Autodesk Inventor part; units mm, degrees
ref_plane "YZ Plane" through (0, 0, 0) normal (1, 0, 0) x (0, 1, 0)
ref_plane "XZ Plane" through (0, 0, 0) normal (0, 1, 0) x (-1, 0, 0)
ref_plane "XY Plane" through (0, 0, 0) normal (0, 0, 1) x (1, 0, 0)
sketch "Sketch1" plane through (0, 0, 0) normal (0, 0, 1) x (1, 0, 0)
  line L0 (-13.9879, -6.06) -> (16.0121, -6.06)
  line L1 (16.0121, -6.06) -> (16.0121, 23.94)
  line L2 (16.0121, 23.94) -> (-13.9879, 23.94)
  line L3 (-13.9879, 23.94) -> (-13.9879, -6.06)
  line L4 (-12.2879, 23.94) -> (-12.2879, -6.06)
  line L5 (-13.9879, -4.36) -> (16.0121, -4.36)
  line L6 (14.3121, -6.06) -> (14.3121, 23.94)
  line L7 (16.0121, 22.24) -> (-13.9879, 22.24)
  point P0 (0, 0)
  point P1 (14.3121, 22.24)
  point P2 (-12.2879, 22.24)
  point P3 (-12.2879, -4.36)
  point P4 (14.3121, -4.36)
  dimension "d1" = 30
  dimension "d3" = 1.7
  dimension "d4" = 1.7
  dimension "d5" = 1.7
  dimension "d6" = 1.7
extrude "Extrusion1" add sketch "Sketch1" against normal blind 129.75
extrude "Extrusion2" cut sketch "Sketch1" against normal blind 403 contours L4 L7 L6 L5
properties part number "Cablecanal Ranurado 30 x 30 L = 403" material "PVC-Piping"
Build history of the part. All positions in model axes, mm. A direction names the side the tool comes from. Give positions to 0.01 mm unless a question says otherwise; leave off trailing zeros. Order: outer loops, then holes, each group sorted by start corner. A loop starts at its lowest first (then second) coordinate and runs counter-clockwise, first axis right, second up. Notation, with made-up numbers: M 15,18.25 L 34,18.25 A25 ccw 34,55.25 Z; hole C 38.25,45 d10. An arc over 180 degrees is marked long. Write item = value, one per line. Start each with the question number.
(1) Probe L1, parallel to Y at x = -5, z = -81; L2, parallel to X at y = 10.25, z = -75.5. List the from-to ranges inside material, lowest first. Write a range as [from, to].
(2) Two-plate mould, pull along X, no slides. Class faces 1 (the flat face through (1, -4.36, -64)), 2 (the flat face through (1, -6.06, -64)), 3 (the flat face through (-13.988, 9, -64)), 4 (the flat face through (1, 22.24, -64)): released by +X, released by -X, zero draft, split by the parting line, or undercut.
(3) Slice it at B-B on y = 12.5. Write the cut outline in (x, z), plus the area to 3 significant figures.
(4) Which spindle directions (+Z, -Z, +X, -X, +Y, -Y) get a long thin tool onto all of the face, cutting with end or side? Do faces 5 (the flat face through (16.012, 9, -64)), 6 (the flat face through (-12.288, 9, -64)). Say none if no direction does.
(5) Slice it at C-C on x = 0.75. Write the cut outline in (y, z).
(6) Pin check, flat tip, straight feed: pin 1 Ø12 at (x, y) = (1, 18) entering from -Z. Stop position of the tip, or through.
(7) Slice it at A-A on z = -23. Write the cut outline in (x, y), plus the area to 3 significant figures.
Responses:
q1.L1 = [-6.06, -4.36], [22.24, 23.94]
q1.L2 = [-13.99, -12.29], [14.31, 16.01]
q2.face_1 = undercut
q2.face_2 = zero draft
q2.face_3 = released by -X
q2.face_4 = undercut
q3.outline = M -13.99,-129.75 L -12.29,-129.75 L -12.29,0 L -13.99,0 Z; M 14.31,-129.75 L 16.01,-129.75 L 16.01,0 L 14.31,0 Z
q3.area = 441 mm2
q4.face_5 = +Z, -Z, +X, +Y, -Y
q4.face_6 = +Z, -Z
q5.outline = M -6.06,-129.75 L -4.36,-129.75 L -4.36,0 L -6.06,0 Z; M 22.24,-129.75 L 23.94,-129.75 L 23.94,0 L 22.24,0 Z
q6.pin_1 = -129.75
q7.outline = M -13.99,-6.06 L 16.01,-6.06 L 16.01,23.94 L -13.99,23.94 Z; hole M -12.29,-4.36 L 14.31,-4.36 L 14.31,22.24 L -12.29,22.24 Z
q7.area = 192 mm2
